CAD build for the part. Positions are in the model's coordinates, mm. Round coordinates to 2 decimals unless told otherwise and drop trailing zeros. Loops run counter-clockwise (first coordinate to the right, second up) from the corner with the lowest first, then second, coordinate; pieces in that order, holes last. Notation, with made-up numbers: M -13,31.5 L 44,31.5 A23 ccw 44,58.5 Z; hole C 0,67.25 d4. An arc over 180 degrees is marked long. Use a Markdown table: item, result. Add a question column.
(1) Wall check: L1, parallel to Y at x = -62, z = -4.5; L2, parallel to X at y = 114, z = -35.5; L3, parallel to Y at x = -168.5, z = -50.5. Give the ranges that are in metal, low to high.
(2) Band-saw the part on A-A, the plane y = 110.5. Write the cut outline in (x, z), and give its area (3 significant figures).
(3) Flat gauge pins, fed straight in: P1, Ø6, axis at x = 124.5, z = -17.5, coming from the -Y side; P2, Ø17, axis at y = -49.5, z = -39.5, coming from the -X side; P3, Ø8, axis at x = -54, z = -9, coming from the +Y side. Where does each tip first touch, or does it go through?
(4) Band-saw the part on C-C, the plane z = -16.5. Write the cut outline in (x, y), and give its area (3 significant figures).
(5) Band-saw the part on B-B, the plane x = -140.5. Write the cut outline in (y, z), and give its area (3 significant figures).
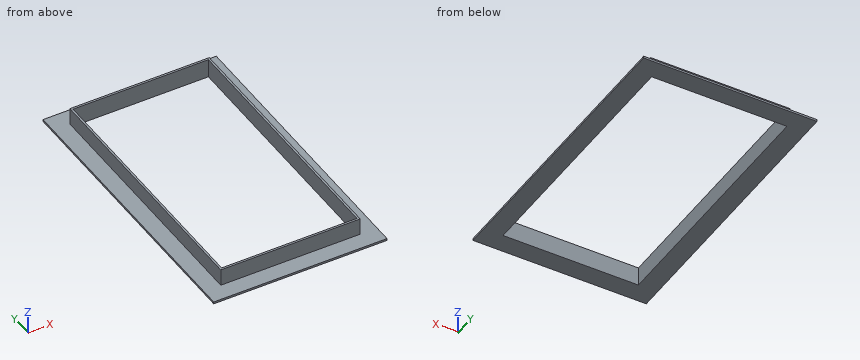
from build123d import *

# Parameters (mm, degrees)
SKETCH054_W            = 400
SKETCH054_H            = 60
PAD003_DEPTH           = 375
SKETCH004_W            = 412
SKETCH004_H            = 50
PAD004_DEPTH           = 381
SKETCH055_W            = 512
SKETCH055_H            = 862
PAD005_DEPTH           = 6
CUT001_PLACEMENT_ANGLE = 180


with BuildPart() as body002:
    # Sketch054 → Pad003 (new body, symmetric)
    with BuildSketch(Plane.XZ):
        with Locations((0, 30)):
            Rectangle(SKETCH054_W, SKETCH054_H)
    extrude(amount=PAD003_DEPTH, both=True)


with BuildPart() as cut001:
    # Sketch004 → Pad004 (new body, symmetric)
    with BuildSketch(Plane.XZ):
        with Locations((0, 25)):
            Rectangle(SKETCH004_W, SKETCH004_H)
    extrude(amount=PAD004_DEPTH, both=True)

    # Sketch055 (on Face3 of Pad004) → Pad005 (join)
    with BuildSketch(Plane(origin=(0, 0, 50), x_dir=(-1, 0, 0), z_dir=(0, 0, 1))):
        Rectangle(SKETCH055_W, SKETCH055_H)
    extrude(amount=PAD005_DEPTH)

    # Cut001: cut Body002
    add(body002.part, mode=Mode.SUBTRACT)


with BuildPart() as cut001_1:
    # Cut001 placement: moved
    add(cut001.part.rotate(Axis((0, 0, 0), (0, 1, 0)), CUT001_PLACEMENT_ANGLE))


solid = cut001_1.part
Return value:
| question | item | result |
|---|---|---|
| 1 | L1 | -381 to -375, 375 to 381 |
| 1 | L2 | -206 to -200, 200 to 206 |
| 1 | L3 | -431 to -375, 375 to 431 |
| 2 | outline | M -256,-56 L -200,-56 L -200,0 L -206,0 L -206,-50 L -256,-50 Z; M 200,-56 L 256,-56 L 256,-50 L 206,-50 L 206,0 L 200,0 Z |
| 2 | area | 1,270 mm^2 |
| 3 | P1 | y = -381 |
| 3 | P2 | x = -206 |
| 3 | P3 | y = 381 |
| 4 | outline | M -206,-381 L 206,-381 L 206,381 L -206,381 Z; hole M -200,-375 L 200,-375 L 200,375 L -200,375 Z |
| 4 | area | 13,900 mm^2 |
| 5 | outline | M -431,-56 L -375,-56 L -375,0 L -381,0 L -381,-50 L -431,-50 Z; M 375,-56 L 431,-56 L 431,-50 L 381,-50 L 381,0 L 375,0 Z |
| 5 | area | 1,270 mm^2 |
